Check sheet for the modelled part. Datum: model origin and axes. Units: mm. A direction names the side the tool comes from. Round coordinates to 2 decimals unless told otherwise and drop trailing zeros. Loops run counter-clockwise (first coordinate to the right, second up) from the corner with the lowest first, then second, coordinate; pieces in that order, holes last. Notation, with made-up numbers: (-26, 51.25) - (29, 51.25) arc R27 cw to (29, 89.25) - close; hole circle Ø3 at (-9.75, 27.5). An arc over 180 degrees is marked (long way). Put each result on its own line as item: value. Start each with the question number.
Item 1: Material ranges on line 1 along Y through (x, z) = (12, 30); line 2 along Z through (x, y) = (6, 18); line 3 along Y through (x, z) = (4.5, 9.75), recorded low to high.
Item 2: Draft check along Y on faces 4 (the flat face through (36.76, 10, 8)), 5 (the cylindrical face through (4.9, 25.85, 9.59)), 6 (the flat face through (-32, 3, 26)). Enter one of: pulls with the +Y half, pulls with the -Y half, needs draft (parallel to the pull), parting line crosses it, or undercut.
Item 3: Section check A-A, the plane x = 32. Record the cut outline in (y, z).
Item 4: Section check B-B, the plane z = -18. Record the cut outline in (x, y), and give its area (3 significant figures).
Item 5: Section check D-D, the plane x = 0. Record the cut outline in (y, z), and give its area (3 significant figures).
Item 6: Tool access check on faces 1 (the cylindrical face through (14.295, 41.435, 10.823)), 2 (the flat face through (14, 44.3, 34)), 3 (the flat face through (12.76, 37, 30)). Record the directions out of +Z, -Z, +X, -X, +Y, -Y that give a thin tool (end or side, any length) a straight path to the whole face; none if there is none.
Item 7: Section check C-C, the plane x = -31.5. Record the cut outline in (y, z), and give its area (3 significant figures).
Item 8: Gauge pin test, flat ends, axial feed: pin 1 Ø1.6 at (x, z) = (6, 4) entering from +Y; pin 2 Ø3 at (x, y) = (4.5, 24) entering from -Z; pin 3 Ø3 at (y, z) = (18.3, 9.75) entering from -X; pin 4 Ø8 at (x, z) = (-34, -1.5) entering from -Y. Record the tip position at first contact, or that the pin passes through.
from build123d import *

# Parameters (mm, degrees)
SKETCH_1_R           = 65
EXTRUDE_1_DEPTH      = 5
SKETCH_2_W           = 6
SKETCH_2_H           = 35
EXTRUDE_2_DEPTH      = 60
FILLET_1_R           = 17.5
SKETCH_3_R           = 16
CUT_EXTRUDE_1_DEPTH  = 5
CHAMFER_1_SIZE       = 1.640243073
CHAMFER_1_SIZE_2     = 0.8
SKETCH_4_R           = 15
CUT_EXTRUDE_2_DEPTH  = 118.234882236
SKETCH_6_W           = 2
SKETCH_6_H           = 6
CUT_EXTRUDE_3_DEPTH  = 118.858124934
SKETCH_8_R           = 1.6
CUT_EXTRUDE_5_DEPTH  = 6
CUT_EXTRUDE_START    = -2
CUT_EXTRUDE_8_DEPTH  = 2.2
SKETCH_11_W          = 25
SKETCH_11_H          = 10.5
EXTRUDE_4_DEPTH      = 7.3
EXTRUDE_5_DEPTH      = 2
FILLET_3_R           = 1
EXTRUDE_6_DEPTH      = 5
SKETCH_14_R          = 1.15
CUT_EXTRUDE_10_DEPTH = 124.023158848
FILLET_2_R           = 0.5
SKETCH_15_R          = 2
CUT_EXTRUDE_11_DEPTH = 10
SKETCH_16_W          = 53.828401117
SKETCH_16_H          = 62.5
CUT_EXTRUDE_12_DEPTH = 2


# Some blends are built 0.0001 mm under size
with BuildPart() as part:
    # 스케치1 → 보스-돌출1 (new body)
    with BuildSketch(Plane(origin=(0, 0, 0), x_dir=(1, 0, 0), z_dir=(0, 1, 0))):
        with Locations(Location((0, 0, 0), (0, 0, 270))):
            Circle(SKETCH_1_R)
    extrude(amount=EXTRUDE_1_DEPTH)

    # 스케치2 → 보스-돌출2 (add)
    with BuildSketch(Plane(origin=(0, 5, 0), x_dir=(1, 0, 0), z_dir=(0, 1, 0))):
        with Locations((5.76, -20)):
            Rectangle(SKETCH_2_W, SKETCH_2_H)
    extrude(amount=EXTRUDE_2_DEPTH)

    # 필렛1
    fillet_1_edges = [part.edges().sort_by_distance(p)[0] for p in [
        (5.76, 65, 2.5),
        (5.76, 65, 37.5),
    ]]
    fillet(fillet_1_edges, radius=FILLET_1_R - 0.0001)  # a hair under: the kernel refuses the full size

    # 스케치3 → 컷-돌출1 (cut)
    with BuildSketch(Plane.ZY.offset(-2.76)):
        with Locations((20, 47.5)):
            Circle(SKETCH_3_R)
    extrude(amount=-CUT_EXTRUDE_1_DEPTH, mode=Mode.SUBTRACT)

    # 모따기1
    # the kernel refuses this chamfer: 1.640243073, 0.8 mm, written as the material it takes off along each edge
    with BuildSketch(Plane(origin=(2.76, 47.5, 20), x_dir=(0, 0, 1), z_dir=(0, -1, 0))) as chamfer_1_piece_1:
        Polygon((16 + CHAMFER_1_SIZE, 0), (16, -CHAMFER_1_SIZE_2), (16, 0), align=None)
    revolve(axis=Axis((2.76, 47.5, 20), (-1, 0, 0)), mode=Mode.SUBTRACT)

    # 스케치4 → 컷-돌출2 (cut, through all)
    with BuildSketch(Plane.ZY.offset(-7.76)):
        with Locations((20, 47.5)):
            Circle(SKETCH_4_R)
    extrude(amount=-CUT_EXTRUDE_2_DEPTH, mode=Mode.SUBTRACT)

    # 스케치6 → 컷-돌출3 (cut, through all)
    with BuildSketch(Plane(origin=(8.76, 0, 0), x_dir=(0, 0, -1), z_dir=(1, 0, 0))):
        with Locations((-3.5, 24.5)):
            Rectangle(SKETCH_6_W, SKETCH_6_H)
    extrude(amount=-CUT_EXTRUDE_3_DEPTH, mode=Mode.SUBTRACT)

    # 스케치8 → 컷-돌출5 (cut)
    with BuildSketch(Plane(origin=(0, 0, 4.5), x_dir=(-1, 0, 0), z_dir=(0, 0, -1))):
        with Locations((-5.76, 24.5)):
            Circle(SKETCH_8_R)
    extrude(amount=-CUT_EXTRUDE_5_DEPTH, mode=Mode.SUBTRACT)

    # 스케치9 → 컷-돌출8 (cut)
    with BuildSketch(Plane(origin=(0, 0, 4.5), x_dir=(-1, 0, 0), z_dir=(0, 0, -1)).offset(CUT_EXTRUDE_START)):
        Polygon((-4.316624327, 27), (-7.203375673, 27), (-8.646751346, 24.5), (-7.203375673, 22), (-4.316624327, 22), (-2.76, 22), (-2.76, 27), align=None)
    extrude(amount=-CUT_EXTRUDE_8_DEPTH, mode=Mode.SUBTRACT)

    # 스케치11 → 보스-돌출4 (add)
    with BuildSketch(Plane(origin=(0, 5, 0), x_dir=(1, 0, 0), z_dir=(0, 1, 0))):
        with Locations((24.26, -7.75)):
            Rectangle(SKETCH_11_W, SKETCH_11_H)
        with Locations((24.26, -32.25)):
            Rectangle(SKETCH_11_W, SKETCH_11_H)
    extrude(amount=EXTRUDE_4_DEPTH)

    # 스케치12 → 보스-돌출5 (add)
    with BuildSketch(Plane(origin=(0, 12.3, 0), x_dir=(1, 0, 0), z_dir=(0, 1, 0))):
        Polygon((16.76, -32.5), (36.76, -32.5), (36.76, -37.5), (11.76, -37.5), (11.76, -27), (16.76, -27), align=None)
        Polygon((11.76, -2.5), (36.76, -2.5), (36.76, -7.5), (16.76, -7.5), (16.76, -13), (11.76, -13), align=None)
    extrude(amount=EXTRUDE_5_DEPTH)

    # 필렛3
    fillet_3_edges = [part.edges().sort_by_distance(p)[0] for p in [
        (36.76, 9.65, 2.5),
        (36.76, 9.65, 37.5),
        (36.76, 8.65, 27),
        (36.76, 8.65, 13),
    ]]
    fillet(fillet_3_edges, radius=FILLET_3_R)

    # 스케치13 → 보스-돌출6 (add)
    with BuildSketch(Plane(origin=(16.76, 0, 0), x_dir=(0, 0, -1), z_dir=(1, 0, 0))):
        with BuildLine():
            Line((-27, 14.3), (-37.5, 14.3))
            Line((-37.5, 14.3), (-37.5, 44.3))
            Line((-37.5, 44.3), (-30.524257694, 44.3))
            ThreePointArc((-30.524257694, 44.3), (-29.151964364, 41.397414624), (-27, 39.014718626))
            Line((-27, 39.014718626), (-27, 14.3))
        make_face()
        with BuildLine():
            Line((-13, 14.3), (-2.5, 14.3))
            Line((-2.5, 14.3), (-2.5, 44.3))
            Line((-2.5, 44.3), (-9.475742306, 44.3))
            ThreePointArc((-9.475742306, 44.3), (-10.848035636, 41.397414624), (-13, 39.014718626))
            Line((-13, 39.014718626), (-13, 14.3))
        make_face()
    extrude(amount=-EXTRUDE_6_DEPTH)

    # 스케치14 → 컷-돌출10 (cut, through all)
    with BuildSketch(Plane(origin=(16.76, 0, 0), x_dir=(0, 0, -1), z_dir=(1, 0, 0))):
        with Locations((-30.25, 18.3)):
            Circle(SKETCH_14_R)
        with Locations((-9.75, 18.3)):
            Circle(SKETCH_14_R)
        with Locations((-9.75, 38.8)):
            Circle(SKETCH_14_R)
        with Locations((-30.25, 38.8)):
            Circle(SKETCH_14_R)
    extrude(amount=-CUT_EXTRUDE_10_DEPTH, mode=Mode.SUBTRACT)

    # 필렛2
    fillet_2_edges = [part.edges().sort_by_distance(p)[0] for p in [
        (26.26, 12.3, 13),
        (16.76, 25.657359313, 13),
        (26.76, 12.3, 7.5),
        (36.76, 13.3, 7.5),
        (36.76, 12.3, 30.25),
        (16.76, 25.657359313, 27),
        (26.76, 12.3, 32.5),
        (36.76, 13.3, 32.5),
        (26.26, 12.3, 27),
        (36.467106781, 12.3, 27.292893219),
        (36.76, 12.3, 9.75),
        (36.467106781, 12.3, 12.707106781),
    ]]
    fillet(fillet_2_edges, radius=FILLET_2_R)

    # 스케치15 → 컷-돌출11 (cut)
    with BuildSketch(Plane.ZY.offset(-2.76)):
        with Locations((9.75, 38.8)):
            Circle(SKETCH_15_R)
        with Locations((30.25, 38.8)):
            Circle(SKETCH_15_R)
        with Locations((9.75, 18.3)):
            Circle(SKETCH_15_R)
        with Locations((30.25, 18.3)):
            Circle(SKETCH_15_R)
    extrude(amount=-CUT_EXTRUDE_11_DEPTH, mode=Mode.SUBTRACT)

    # 스케치16 → 컷-돌출12 (cut)
    with BuildSketch(Plane(origin=(0, 5, 0), x_dir=(1, 0, 0), z_dir=(0, 1, 0))):
        with Locations((-38.085799442, -33.75)):
            Rectangle(SKETCH_16_W, SKETCH_16_H)
    extrude(amount=-CUT_EXTRUDE_12_DEPTH, mode=Mode.SUBTRACT)


solid = part.part
Check result:
1. line 1: 0 to 16.32, 20.28 to 36.82, 40.78 to 42.92
1. line 2: 2.5 to 7.77, 11.73 to 28.27, 32.23 to 37.5
1. line 3: 0 to 16.3, 20.3 to 23.51, 25.49 to 35.21, 59.79 to 61.68
2. face 4: needs draft
2. face 5: undercut
2. face 6: pulls with the +Y half
3. outline: (0, -56.58) - (5, -56.58) - (5, 2.5) - (14.3, 2.5) - (14.3, 7.5) - (12.8, 7.5) arc R0.5 cw to (12.3, 8) - (12.3, 12.5) arc R0.5 ccw to (11.8, 13) - (5, 13) - (5, 27) - (11.8, 27) arc R0.5 ccw to (12.3, 27.5) - (12.3, 32) arc R0.5 cw to (12.8, 32.5) - (14.3, 32.5) - (14.3, 37.5) - (5, 37.5) - (5, 56.58) - (0, 56.58) - close
4. outline: (-62.46, 0) - (62.46, 0) - (62.46, 5) - (-62.46, 5) - close
4. area: 625 mm²
5. outline: (0, -65) - (5, -65) - (5, 65) - (0, 65) - close
5. area: 650 mm²
6. face 1: +X, -X, +Y
6. face 2: +Z, -Z, +X, +Y
6. face 3: -X
7. outline: (0, -56.86) - (5, -56.86) - (5, 2.5) - (3, 2.5) - (3, 56.86) - (0, 56.86) - close
7. area: 460 mm²
8. pin 1: y = 56.17
8. pin 2: z = 4.5
8. pin 3: x = 12.76
8. pin 4: y = 0
